Drawing for the job (mm, zero at the part's lowest x, y, z). Coordinates: 2 decimals unless noted, no trailing zeros. Loops run counter-clockwise (first coordinate to the right, second up) from the corner with the lowest first, then second, coordinate; pieces in that order, holes last. Notation, with made-up numbers: (34, 4) - (54, 4) arc R10 cw to (54, 21) - close; hole circle Ø2 at (-28.75, 61.5). An arc over 180 degrees is marked (long way). One line per item, written item: value.
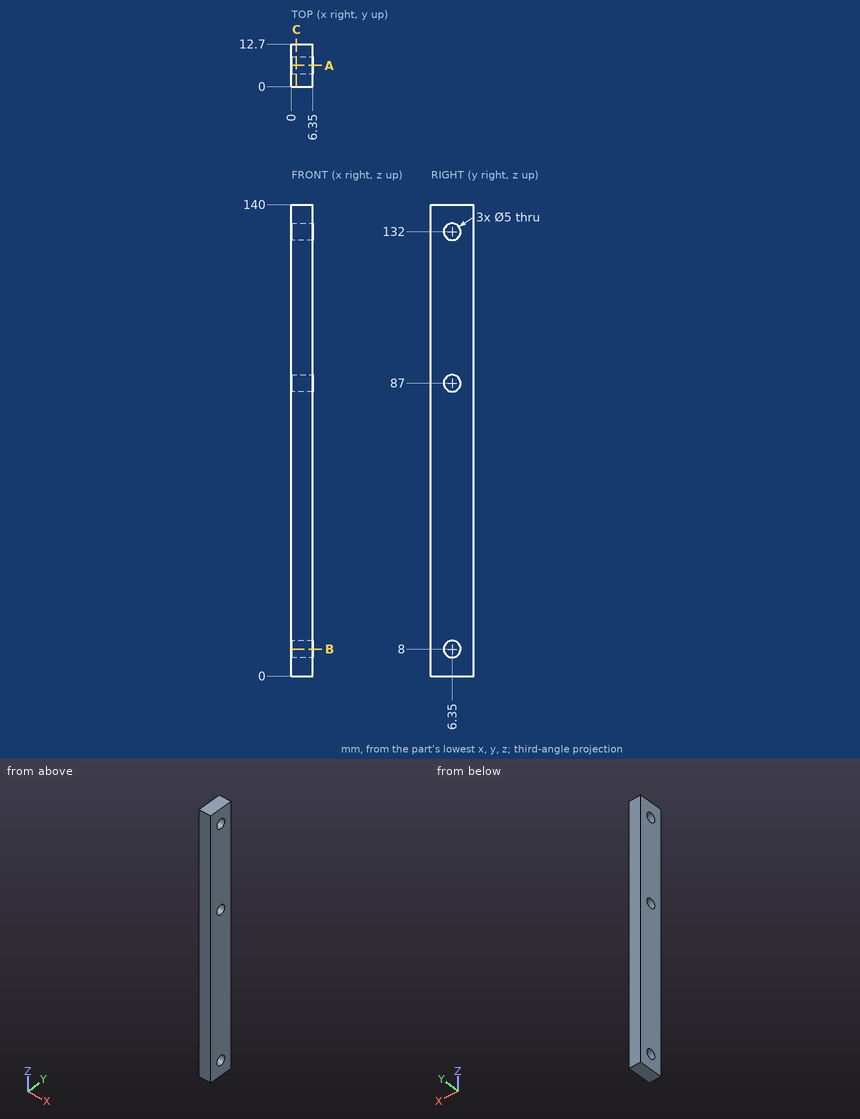
Item 1: Cut at C-C, the plane x = 1.5. Write the cut outline in (y, z), then the cut area to 3 significant figures.
Check result:
outline: (0, 0) - (12.7, 0) - (12.7, 140) - (0, 140) - close; hole circle Ø5 at (6.35, 8); hole circle Ø5 at (6.35, 87); hole circle Ø5 at (6.35, 132)
area: 1,720 mm^2
Item 2: Cut at A-A, the plane y = 6.35. Write the cut outline in (x, z).
Check result:
outline: (0, 0) - (6.35, 0) - (6.35, 5.5) - (0, 5.5) - close; (0, 10.5) - (6.35, 10.5) - (6.35, 84.5) - (0, 84.5) - close; (0, 89.5) - (6.35, 89.5) - (6.35, 129.5) - (0, 129.5) - close; (0, 134.5) - (6.35, 134.5) - (6.35, 140) - (0, 140) - close
Item 3: Probe probe 1 along Y at (x, z) = (2.25, 132); probe 2 along Z at (x, y) = (3.5, 6); probe 3 along Z at (x, y) = (3, 7.5). List the from-to ranges inside material, lowest first. Write a range as from..to.
Check result:
probe 1: y = 0..3.85, 8.85..12.7
probe 2: z = 0..5.52, 10.48..84.52, 89.48..129.52, 134.48..140
probe 3: z = 0..5.78, 10.22..84.78, 89.22..129.78, 134.22..140
Item 4: Cut at B-B, the plane z = 8. Write the cut outline in (x, y), then the cut area to 3 significant figures.
Check result:
outline: (0, 0) - (6.35, 0) - (6.35, 3.85) - (0, 3.85) - close; (0, 8.85) - (6.35, 8.85) - (6.35, 12.7) - (0, 12.7) - close
area: 48.9 mm^2
Item 5: Drop a flat-ended pin along its axis: P1, Ø1.5, axis at x = 3, z = 78, coming from the -Y side. Give the stop position or say it passes through.
Check result:
P1: stops at y = 0
